Answer from the drawing. Dimensions are ordinates in mm from the lowest x, y and z of the part. A direction names the side the tool comes from. Give positions to 0.01 mm unless a question says otherwise; leave off trailing zeros. Write each loop counter-clockwise with the first axis right and the second up, starting at its lowest first coordinate (ties: lowest second). Pieces come first, ordered by that corner, then holes. Notation, with made-up numbers: M 4,17 L 28,17 A20 cw 28,50 Z; hole C 80,-22 d3. An arc over 180 degrees is marked long. Write each question's results on one line, items separated by ' | '. Start each with the question number.
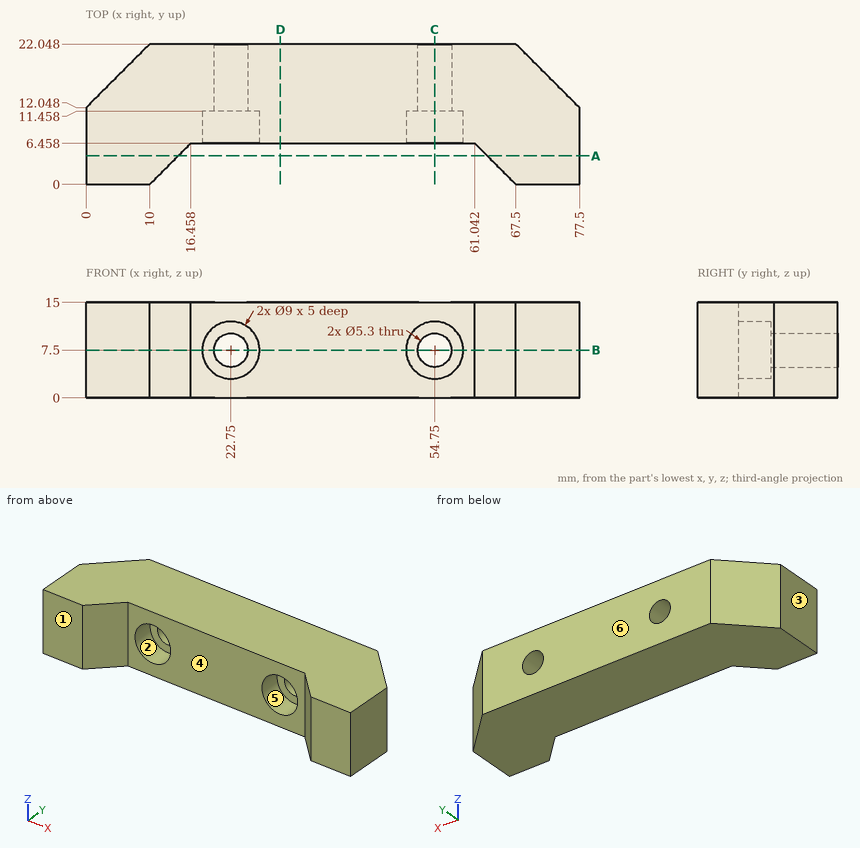
Item 1: Section C-C, the plane x = 54.75 is taken. Determine the outline of the cut face in (y, z), then the cut area to 3 significant figures.
Item 2: Section A-A, the plane y = 4.5 is taken. Determine the outline of the cut face in (x, z), then the cut area to 3 significant figures.
Item 3: Determine the mould class of the marked faces 1, 2 and 3 for opening direction X: +X half, -X half, draft (parallel to the pull), parting line (faces both ways), or undercut.
Item 4: Given P1, Ø6, axis at x = 22.75, z = 7.5, coming from the -Y side; P2, Ø3, axis at y = 14.5, z = 11.5, coming from the -X side; P3, Ø5, axis at x = 54.75, z = 7.5, coming from the -Y side, each flat-ended and moving along its own axis, determine where each tip first touches the part or whether it passes through.
Item 5: Section D-D, the plane x = 30.5 is taken. Determine the outline of the cut face in (y, z).
Item 6: For the marked faces 4, 5 and 6, determine the directions among +Z, -Z, +X, -X, +Y, -Y from which every point of the face is accessible in a straight line to the end or side of a thin tool.
Item 7: Straight lines are drawn through the part: line 1 (Z direction, x = 54.75, y = 9.05); line 2 (Z direction, x = 54.75, y = 18.5); line 3 (X direction, y = 10.5, z = 11.25). For each, find the intervals that lie inside material, in ascending order.
Item 8: Section B-B, the plane z = 7.5 is taken. Determine the outline of the cut face in (x, y).
Worked out:
1) outline: M 6.46,0 L 22.05,0 L 22.05,4.85 L 11.46,4.85 L 11.46,3 L 6.46,3 Z; M 6.46,12 L 11.46,12 L 11.46,10.15 L 22.05,10.15 L 22.05,15 L 6.46,15 Z | area: 133 mm²
2) outline: M 0,0 L 14.5,0 L 14.5,15 L 0,15 Z; M 63,0 L 77.5,0 L 77.5,15 L 63,15 Z | area: 435 mm²
3) face 1: draft | face 2: undercut | face 3: -X half
4) P1: stops at y = 11.46 | P2: stops at x = 0.95 | P3: passes through
5) outline: M 6.46,0 L 22.05,0 L 22.05,15 L 6.46,15 Z
6) face 4: +Z, -Z, -Y | face 5: -Y | face 6: +Z, -Z, +X, -X, +Y
7) line 1: z = 0 to 3, 12 to 15 | line 2: z = 0 to 4.85, 10.15 to 15 | line 3: x = 0 to 20.26, 25.24 to 52.26, 57.24 to 77.5
8) outline: M 0,0 L 10,0 L 16.46,6.46 L 18.25,6.46 L 18.25,11.46 L 20.1,11.46 L 20.1,22.05 L 10,22.05 L 0,12.05 Z; M 25.4,11.46 L 27.25,11.46 L 27.25,6.46 L 50.25,6.46 L 50.25,11.46 L 52.1,11.46 L 52.1,22.05 L 25.4,22.05 Z; M 57.4,11.46 L 59.25,11.46 L 59.25,6.46 L 61.04,6.46 L 67.5,0 L 77.5,0 L 77.5,12.05 L 67.5,22.05 L 57.4,22.05 Z
